Verification items for the finished model (mm, model axes). A direction names the side the tool comes from. Coordinates: 2 decimals unless noted, no trailing zeros. Loops run counter-clockwise (first coordinate to the right, second up) from the corner with the lowest first, then second, coordinate; pieces in that order, holes last. Notation, with made-up numbers: (74, 64.25) -> (102, 64.25) arc R11 cw to (102, 70.25) -> close; hole circle Ø8 at (39.25, -29). An arc over 180 degrees is marked (long way). Answer as a JSON object with one key per item and string values. Group by question number.
Q1. Cross-section at A-A on z = 13.25. Record the boundary of the cut face in (x, y), and give its area (3 significant figures).
Q2. Cross-section at C-C on z = -8. Record the boundary of the cut face in (x, y).
Q3. Cross-section at B-B on y = -9.5. Record the boundary of the cut face in (x, z), and give its area (3 significant figures).
Q4. Set-up check for faces 1 (the cylindrical face through (0.8, -9, -12.1)), 2 (the flat face through (0, -11, 15)), 3 (the cylindrical face through (0.08, -5.99, 15.75)), 4 (the flat face through (0, -9, -10.5)), 5 (the flat face through (-7.29, -4.82, 13.26)): record each of +Z, -Z, +X, -X, +Y, -Y from which the full face is reachable in a straight line by a thin tool's end or side.
Q5. Scan lines: L1, parallel to Z at x = 0, y = -8.15; L2, parallel to X at y = 4.5, z = 0; L3, parallel to Y at x = -3, z = -14.5. Record each from-to range of solid material in increasing order.
Q6. Gauge pin test, flat ends, axial feed: pin 1 Ø2.5 at (x, z) = (0, 13.25) entering from -Y; pin 2 Ø6.5 at (x, z) = (0.5, 1.5) entering from -Y; pin 3 Ø1.5 at (x, z) = (-2.5, 7.5) entering from +Y; pin 4 Ø1.8 at (x, z) = (0, 0) entering from +Y. Record the tip position at first contact, or that the pin passes through.
Q7. Release check for a two-part mould opening along X. For faces 6 (the flat face through (7.59, -0.51, 11.36)), 7 (the cylindrical face through (-1.46, -4.51, -6.59)), 8 (the flat face through (-7.372, -4.819, -13.073)) record: released by +X, released by -X, zero draft, split by the parting line, or undercut.
```python
from build123d import *

# Parameters (mm, degrees)
CUT_EXTRUDE1_DEPTH  = 12
SKETCH5_W           = 24
SKETCH5_H           = 21
CUT_EXTRUDE3_DEPTH  = 6
FILLET1_R           = 0.5
FILLET3_R           = 0.5
CHAMFER2_SIZE       = 1
SKETCH12_R          = 1.4
CUT_EXTRUDE7_DEPTH  = 6
SKETCH13_R          = 7.375
CUT_EXTRUDE8_DEPTH  = 2
SKETCH14_R          = 7.375
SKETCH14_R_2        = 6.75
BOSS_EXTRUDE1_DEPTH = 1


with BuildPart() as part:
    # Sketch2 → Revolve1 (revolve)
    with BuildSketch(Plane(origin=(0, 0, 0), x_dir=(0, 0, -1), z_dir=(1, 0, 0))):
        Polygon((-2.5, 0), (-21.75, 0), (-21.75, -11), (-8.75, -11), (-8.75, -7), (-15.75, -7), (-15.75, -5), (-1.5, -5), (-1.5, 6), (-1.5, 7.616444111), (-2.5, 7.616444111), (-2.5, 6), (-3, 5), (-2.5, 5), (-2.5, 2), (-3, 1), (-2.5, 1), align=None)
    revolve(axis=Axis((0, 7.880012575, 0), (0, -1, 0)))

    # Sketch3 → Cut-Extrude1 (cut, through all)
    with BuildSketch(Plane(origin=(0, 0, 0), x_dir=(1, 0, 0), z_dir=(0, 1, 0))):
        with BuildLine():
            ThreePointArc((-10.990322793, -4.817966886), (-12, 0), (-10.990322793, 4.817966886))
            Line((-10.990322793, 4.817966886), (-5, 18.48256498))
            ThreePointArc((-5, 18.48256498), (-2.986475006, 20.860711972), (-2.4e-08, 21.75))
            ThreePointArc((-2.4e-08, 21.75), (-21.75, -1.1e-08), (-2e-09, -21.75))
            ThreePointArc((-2e-09, -21.75), (-2.986474997, -20.860711978), (-5, -18.48256498))
            Line((-5, -18.48256498), (-10.990322793, -4.817966886))
        make_face()
        with BuildLine():
            ThreePointArc((21.75, 0), (15.379572482, 15.379572499), (-2.4e-08, 21.75))
            ThreePointArc((-2.4e-08, 21.75), (2.986474986, 20.860711985), (5, 18.48256498))
            Line((5, 18.48256498), (10.990322793, 4.817966886))
            ThreePointArc((10.990322793, 4.817966886), (12, 0), (10.990322793, -4.817966886))
            Line((10.990322793, -4.817966886), (5, -18.48256498))
            ThreePointArc((5, -18.48256498), (2.986474995, -20.860711979), (-2e-09, -21.75))
            ThreePointArc((-2e-09, -21.75), (15.37957249, -15.379572492), (21.75, 0))
        make_face()
    extrude(amount=-CUT_EXTRUDE1_DEPTH, mode=Mode.SUBTRACT)

    # Sketch5 → Cut-Extrude3 (cut)
    with BuildSketch(Plane.XZ.offset(11)):
        Rectangle(SKETCH5_W, SKETCH5_H)
    extrude(amount=-CUT_EXTRUDE3_DEPTH, mode=Mode.SUBTRACT)

    # Fillet1
    fillet1_edges = [part.edges().sort_by_distance(p)[0] for p in [
        (8.49941803, -9, 10.5),
        (-8.49941803, -9, 10.5),
        (-8.49941803, -9, -10.5),
        (-6.894608136, -6, -14.160751345),
        (-6.894608136, -6, 14.160751345),
        (6.894608136, -6, -14.160751345),
        (6.894608136, -6, 14.160751345),
        (8.49941803, -9, -10.5),
    ]]
    fillet(fillet1_edges, radius=FILLET1_R)

    # Fillet3
    fillet3_edges = [part.edges().sort_by_distance(p)[0] for p in [
        (0, 0, -2.5),
    ]]
    fillet(fillet3_edges, radius=FILLET3_R)

    # Chamfer2
    chamfer2_edges = [part.edges().sort_by_distance(p)[0] for p in [
        (0, 0, 21.75),
        (-7.995161396, 0, 11.650265933),
        (-12, 0, 0),
        (-7.995161396, 0, -11.650265933),
        (0, 0, -21.75),
        (7.995161396, 0, 11.650265933),
        (7.995161396, 0, -11.650265933),
        (12, 0, 0),
    ]]
    chamfer(chamfer2_edges, length=CHAMFER2_SIZE)

    # Sketch12 → Cut-Extrude7 (cut)
    with BuildSketch(Plane.XZ.offset(11)):
        with Locations((0, -13.25)):
            Circle(SKETCH12_R)
        with Locations((0, 13.25)):
            Circle(SKETCH12_R)
    extrude(amount=-CUT_EXTRUDE7_DEPTH, mode=Mode.SUBTRACT)

    # Sketch13 → Cut-Extrude8 (cut)
    with BuildSketch(Plane.XZ.offset(5)):
        Circle(SKETCH13_R)
    extrude(amount=-CUT_EXTRUDE8_DEPTH, mode=Mode.SUBTRACT)


with BuildPart() as body_2:
    # Sketch14 → Boss-Extrude1 (new body)
    with BuildSketch(Plane.XZ.offset(5)):
        Circle(SKETCH14_R)
        Circle(SKETCH14_R_2, mode=Mode.SUBTRACT)
    extrude(amount=-BOSS_EXTRUDE1_DEPTH)


with BuildPart() as part_1:
    add(part.part)

    # Combine1: union body 2
    add(body_2.part)


solid = part_1.part
```
Computed values:
{
 "1": {"outline": "(-7.29, -11) -> (-1.4, -11) -> (-1.4, -7) -> (-7.29, -7) -> close; (-7.29, -5) -> (7.29, -5) -> (7.29, -1) -> (6.2, 0) -> (-6.2, 0) -> (-7.29, -1) -> close; (1.4, -11) -> (7.29, -11) -> (7.29, -7) -> (1.4, -7) -> close", "area": "119 mm²"},
 "2": {"outline": "(-9.6, -5) -> (9.6, -5) -> (9.6, -1) -> (8.5, 0) -> (-8.5, 0) -> (-9.6, -1) -> close"},
 "3": {"outline": "(-8.19, -11.2) -> (-5, -18.48) arc R5.46 ccw to (5, -18.48) -> (8.19, -11.2) arc R0.5 ccw to (7.73, -10.5) -> (-7.73, -10.5) arc R0.5 ccw to start; (-8.19, 11.2) arc R0.5 ccw to (-7.73, 10.5) -> (7.73, 10.5) arc R0.5 ccw to (8.19, 11.2) -> (5, 18.48) arc R5.46 ccw to (-5, 18.48) -> close; hole circle Ø2.8 at (0, -13.25); hole circle Ø2.8 at (0, 13.25)", "area": "250 mm²"},
 "4": {"face 1": "-Y", "face 2": "+Z, -Z, +X, -X, -Y", "face 3": "none", "face 4": "+X, -X, -Y", "face 5": "+Z, -X, +Y, -Y"},
 "5": {"L1": "z = -21.75 to -14.65, -11.85 to -10.5, 10.5 to 11.85, 14.65 to 21.75", "L2": "x = -2.5 to -1.5, 1.5 to 2.5", "L3": "y = -11 to -7, -5 to 0"},
 "6": {"pin 1": "stops at y = -5", "pin 2": "stops at y = -3", "pin 3": "stops at y = 0", "pin 4": "passes through"},
 "7": {"face 6": "released by +X", "face 7": "undercut", "face 8": "released by -X"}
}
